Input: part model. Units: mm. Frame: model coordinates. A direction names the side the tool comes from. Round coordinates to 2 decimals unless told otherwise and drop trailing zeros. Write each loop counter-clockwise with the first axis right and the second up, starting at its lowest first coordinate (ties: lowest second). Pieces come first, ordered by that corner, then holes. Notation, with made-up numbers: M -28.5,-27.75 L 15.5,-27.75 A19 ccw 15.5,7.25 Z; hole C 88,-30 d7. An arc over 180 degrees is marked long. Answer as CSV lines item,"result". Start each with the question number.
```python
from build123d import *

# Parameters (mm, degrees)
BOSS_EXTRUDE1_DEPTH = 30
CUT_EXTRUDE1_DEPTH  = 35
FILLET1_R           = 60
SKETCH6_R           = 25
CUT_EXTRUDE2_DEPTH  = 31
CUT_EXTRUDE3_START  = -27
SKETCH7_W           = 60
SKETCH7_H           = 60
CUT_EXTRUDE3_DEPTH  = 27
SKETCH8_W           = 27.5
SKETCH8_H           = 50
CUT_EXTRUDE4_DEPTH  = 21


with BuildPart() as part:
    # Sketch3 → Boss-Extrude1 (new body)
    with BuildSketch(Plane.XY):
        with BuildLine():
            Line((-57.5, 0), (-57.5, 150))
            ThreePointArc((-57.5, 150), (0, 207.5), (57.5, 150))
            Line((57.5, 150), (57.5, 0))
            ThreePointArc((57.5, 0), (0, -57.5), (-57.5, 0))
        make_face()
    extrude(amount=BOSS_EXTRUDE1_DEPTH)

    # Sketch4 → Cut-Extrude1 (cut)
    with BuildSketch(Plane(origin=(0, 0, 0), x_dir=(-1, 0, 0), z_dir=(0, 0, -1))):
        with BuildLine():
            ThreePointArc((-57.5, 150), (-52.261362401, 126.020842383), (-37.5, 106.411010565))
            Line((-37.5, 106.411010565), (-37.5, 43.588989435))
            ThreePointArc((-37.5, 43.588989435), (-52.261362401, 23.979157617), (-57.5, 0))
            Line((-57.5, 0), (-57.5, 150))
        make_face()
        with BuildLine():
            ThreePointArc((57.5, 0), (52.261362401, 23.979157617), (37.5, 43.588989435))
            Line((37.5, 43.588989435), (37.5, 106.411010565))
            ThreePointArc((37.5, 106.411010565), (52.261362401, 126.020842383), (57.5, 150))
            Line((57.5, 150), (57.5, 0))
        make_face()
    extrude(amount=-CUT_EXTRUDE1_DEPTH, mode=Mode.SUBTRACT)

    # Fillet1
    fillet1_edges = [part.edges().sort_by_distance(p)[0] for p in [
        (37.5, 106.411010565, 15),
        (37.5, 43.588989435, 15),
        (-37.5, 43.588989435, 15),
        (-37.5, 106.411010565, 15),
    ]]
    fillet(fillet1_edges, radius=FILLET1_R)

    # Sketch6 → Cut-Extrude2 (cut, through all)
    with BuildSketch(Plane.XY.offset(30)):
        with Locations((0, 150)):
            Circle(SKETCH6_R)
    extrude(amount=-CUT_EXTRUDE2_DEPTH, mode=Mode.SUBTRACT)

    # Sketch7 → Cut-Extrude3 (cut)
    with BuildSketch(Plane.XY.offset(30).offset(CUT_EXTRUDE3_START)):
        with Locations((0, 150)):
            Rectangle(SKETCH7_W, SKETCH7_H)
    extrude(amount=CUT_EXTRUDE3_DEPTH, mode=Mode.SUBTRACT)

    # Sketch8 → Cut-Extrude4 (cut)
    with BuildSketch(Plane.XY.offset(30)):
        with Locations((-43.75, 150)):
            Rectangle(SKETCH8_W, SKETCH8_H)
    extrude(amount=-CUT_EXTRUDE4_DEPTH, mode=Mode.SUBTRACT)


solid = part.part
```
Item 1: Cut plane A-A, the plane x = 0. Return loops of the section in (y, z), plus the area to 3 significant figures.
Item 2: Draft query along X for faces 6 (the face through (-37.5, 75, 15)), 7 (the face through (0, 177, 3)), 8 (the face through (37.5, 75, 15)), 9 (the face through (-44, 150, 9)). Return one class per face: +X half, -X half, draft (parallel to the pull), parting line (faces both ways), or undercut.
Item 3: Cut plane D-D, the plane y = -14.5. Return loops of the section in (x, z).
Item 4: Cut plane B-B, the plane z = 16.5. Return loops of the section in (x, y).
Item 5: Cut plane C-C, the plane y = 115. Return loops of the section in (x, z), plus the area to 3 significant figures.
Item 6: Line query: line 1 (Y direction, x = -46.5, z = 11.25); line 2 (Y direction, x = 0, z = 1.45); line 3 (Y direction, x = -51, z = 27.25). Output: solid intervals per line, ascending. Write a range as [from, to].
Item 7: Pin query (flat end, axial travel): pin 1 Ø9.5 at (y, z) = (70.5, 11.5) entering from -X; pin 2 Ø15 at (y, z) = (72.5, 16.5) entering from +X; pin 3 Ø1.5 at (x, z) = (-11.5, 8) entering from +Y. Return the tip coordinate at first contact, or that it passes through.
Item 8: Access query for faces 1 (the face through (-41, 125, 20)), 2 (the face through (-3.255, 174.787, 1.521)), 3 (the face through (-40.038, 101.691, 15.21)), 4 (the face through (-30, 150, 7)), 5 (the face through (40.183, 47.833, 15.21)). Directions: +Z, -Z, +X, -X, +Y, -Y. A direction counts if a zero-diameter tool reaches every point of the face in a straight line with its end or side. Return the directions, or none.
Results list:
1,outline,"M -57.5,0 L 125,0 L 125,3 L 120,3 L 120,30 L -57.5,30 Z; M 175,0 L 207.5,0 L 207.5,30 L 180,30 L 180,3 L 175,3 Z"
1,area,"6,180 mm²"
2,face 6,"-X half"
2,face 7,"undercut"
2,face 8,"+X half"
2,face 9,"draft"
3,outline,"M -55.64,0 L 55.64,0 L 55.64,30 L -55.64,30 Z"
4,outline,"M -51.78,125 A57.5 ccw -47.71,117.91 A60 cw -37.5,84.43 L -37.5,65.57 A60 cw -47.71,32.09 A57.5 ccw long 47.71,32.09 A60 cw 37.5,65.57 L 37.5,84.43 A60 cw 47.71,117.91 A57.5 ccw long -51.78,175 L -30,175 L -30,180 L 30,180 L 30,120 L -30,120 L -30,125 Z"
5,outline,"M -45.87,0 L 45.87,0 L 45.87,30 L -45.87,30 Z"
5,area,"2,750 mm²"
6,line 1,"[-33.82, 33.97], [116.03, 125], [175, 183.82]"
6,line 2,"[-57.5, 125], [175, 207.5]"
6,line 3,"[-26.56, 26.56], [123.44, 125], [175, 176.56]"
7,pin 1,"x = -37.5"
7,pin 2,"x = 37.5"
7,pin 3,"y = 206.49"
8,face 1,"+Z, -X"
8,face 2,"+Z, -Z"
8,face 3,"+Z, -Z, -X"
8,face 4,"+Z"
8,face 5,"+Z, -Z, +X"
